Source: CAD feature listing. Evaluate the final solid. Frame: model axes, mm. A direction names the side the tool comes from. Round coordinates to 2 decimals unless told otherwise and drop trailing zeros. Loops run counter-clockwise (first coordinate to the right, second up) from the corner with the lowest first, then second, coordinate; pieces in that order, holes last.
(1) Section A-A, the plane x = 2. Return the cut outline in (y, z), plus the area to 3 significant figures.
(2) Mould query, pull axis Z, two halves, no side actions, for faces 1 (the flat face through (12, 35, 32)), 2 (the flat face through (26, 0, 17)), 3 (the flat face through (25, 35, 17)), 4 (the flat face through (15, 35, 0)). Classes: pulls with the +Z half, pulls with the -Z half, needs draft (parallel to the pull), parting line crosses it, or undercut.
(3) Set-up query: faces 5 (the flat face through (0, 35, 33)), 6 (the flat face through (12, 35, 2)). Return all of +Z, -Z, +X, -X, +Y, -Y with unobstructed straight access to the full face (end or side cutting, diameter ignored); none if empty.
(4) Material intervals for probe 1 along Y at (x, z) = (15, 0.8); probe 2 along Z at (x, y) = (6.75, 43); probe 3 along X at (y, z) = (56, 1.15), sorted ascending.
(5) First-contact query: pin 1 Ø1 at (y, z) = (43, 6.5) entering from -X. Flat tip, straight axial feed; report the tip coordinate or a pass-through.
(6) Section D-D, the plane z = 7.5. Return the cut outline in (x, y), plus the area to 3 significant figures.
(7) Section B-B, the plane y = 39. Return the cut outline in (x, z).
(8) Section C-C, the plane x = 13. Return the cut outline in (y, z).
```python
from build123d import *

# Parameters (mm, degrees)
F0_W     = 30
F0_H     = 70
F1_DEPTH = 2
F2_W     = 5
F2_H     = 70
F3_DEPTH = 30
F4_W     = 30
F4_H     = 70
F5_DEPTH = 2
F7_DEPTH = 5


with BuildPart() as f1:
    # F0 (on Top) → F1 (new body)
    with BuildSketch(Plane.XY):
        with Locations((15, 35)):
            Rectangle(F0_W, F0_H)
    extrude(amount=F1_DEPTH)

    # F2 (on face) → F3 (join)
    with BuildSketch(Plane.XY.offset(2)):
        with Locations((27.5, 35)):
            Rectangle(F2_W, F2_H)
    extrude(amount=F3_DEPTH)

    # F4 (on face) → F5 (join)
    with BuildSketch(Plane.XY.offset(32)):
        with Locations((15, 35)):
            Rectangle(F4_W, F4_H)
    extrude(amount=F5_DEPTH)

    # F6 (on face) → F7 (cut)
    with BuildSketch(Plane(origin=(0, 0, 0), x_dir=(1, 0, 0), z_dir=(0, 0, -1))):
        with BuildLine():
            ThreePointArc((18, -14), (17.12132, -11.87868), (15, -11))
            Line((15, -11), (15, -14))
            Line((15, -14), (15, -17))
            ThreePointArc((15, -17), (17.12132, -16.12132), (18, -14))
        make_face()
        with BuildLine():
            ThreePointArc((18, -56), (17.12132, -53.87868), (15, -53))
            ThreePointArc((15, -53), (12.87868, -58.12132), (18, -56))
        make_face()
        with BuildLine():
            Line((15, -14), (15, -11))
            ThreePointArc((15, -11), (12, -14), (15, -17))
            Line((15, -17), (15, -14))
        make_face()
    extrude(amount=-F7_DEPTH, mode=Mode.SUBTRACT)


solid = f1.part
```
Output values:
1. outline: (0, 0) - (70, 0) - (70, 2) - (0, 2) - close; (0, 32) - (70, 32) - (70, 34) - (0, 34) - close
1. area: 280 mm2
2. face 1: undercut
2. face 2: needs draft
2. face 3: undercut
2. face 4: pulls with the -Z half
3. face 5: +Z, -Z, -X, +Y, -Y
3. face 6: -X, +Y, -Y
4. probe 1: y = 0 to 11, 17 to 53, 59 to 70
4. probe 2: z = 0 to 2, 32 to 34
4. probe 3: x = 0 to 12, 18 to 30
5. pin 1: stops at x = 25
6. outline: (25, 0) - (30, 0) - (30, 70) - (25, 70) - close
6. area: 350 mm2
7. outline: (0, 0) - (30, 0) - (30, 34) - (0, 34) - (0, 32) - (25, 32) - (25, 2) - (0, 2) - close
8. outline: (0, 0) - (11.76, 0) - (11.76, 2) - (0, 2) - close; (0, 32) - (70, 32) - (70, 34) - (0, 34) - close; (16.24, 0) - (53.76, 0) - (53.76, 2) - (16.24, 2) - close; (58.24, 0) - (70, 0) - (70, 2) - (58.24, 2) - close
